from build123d import *

# Parameters (mm, degrees)
SKETCH_1_R      = 2.5
EXTRUDE_1_DEPTH = 80
SKETCH_2_R      = 2
EXTRUDE_2_DEPTH = 5
EXTRUDE_START   = 5
SKETCH_3_R      = 2
EXTRUDE_3_DEPTH = 5


with BuildPart() as part:
    # 草图1 → 凸台-拉伸1 (new body)
    with BuildSketch(Plane.XY):
        with Locations((-0.6401844, 5.281521297)):
            Circle(SKETCH_1_R)
    extrude(amount=EXTRUDE_1_DEPTH)

    # 草图2 → 凸台-拉伸2 (add)
    with BuildSketch(Plane.XY.offset(80)):
        with Locations((-0.6401844, 5.281521297)):
            Circle(SKETCH_2_R)
    extrude(amount=EXTRUDE_2_DEPTH)

    # 草图3 → 凸台-拉伸3 (add)
    with BuildSketch(Plane(origin=(0, 0, 0), x_dir=(-1, 0, 0), z_dir=(0, 0, -1)).offset(EXTRUDE_START)):
        with Locations(Location((0.6401844, 5.281521297, 0), (0, 0, 180))):
            Circle(SKETCH_3_R)
    extrude(amount=-EXTRUDE_3_DEPTH)


solid = part.part
Geometry: final body of the model. Coordinates: model frame, mm. A direction names the side the tool comes from. Give positions to 0.01 mm unless a question says otherwise; leave off trailing zeros. Write each loop counter-clockwise with the first axis right and the second up, starting at its lowest first coordinate (ties: lowest second). Pieces come first, ordered by that corner, then holes.
(1) First-contact query: P1, Ø2, axis at x = -2.5, z = 54.5, coming from the -Y side; P2, Ø1.5, axis at x = -2.5, z = 22, coming from the -Y side; P3, Ø1, axis at x = -1.5, z = 43.5, coming from the -Y side. Flat tips, straight axial feed; report the tip coordinate or a pass-through.
(2) Cut plane C-C, the plane z = 27. Return loops of the section in (x, y).
(3) Ray query, line 1 (X direction, y = 3.8, z = 61); line 2 (Z direction, x = -1.75, y = 7.05); line 3 (Y direction, x = 0.85, z = 57). Return the intervals inside material, ascending.
(4) Cut plane A-A, the plane x = -0.25. Return loops of the section in (y, z).
(5) Cut plane B-B, the plane y = 4.1. Return loops of the section in (x, z), then the cut area to 3 significant figures.
(6) Access query for faces 1 (the flat face through (-1, 5, 85)), 2 (the flat face through (-2, 7, 80)), 3 (the cylindrical face through (0.283, 7.056, -2.535)). Directions: +Z, -Z, +X, -X, +Y, -Y. A direction counts if a zero-diameter tool reaches every point of the face in a straight line with its end or side. Return the directions, or none.
Values follow:
1. P1: stops at y = 2.93
1. P2: stops at y = 3.04
1. P3: stops at y = 2.81
2. outline: circle Ø5 at (-0.64, 5.28)
3. line 1: x = -2.65 to 1.37
3. line 2: z = 0 to 80
3. line 3: y = 3.27 to 7.29
4. outline: (2.81, 0) - (3.32, 0) - (3.32, -5) - (7.24, -5) - (7.24, 0) - (7.75, 0) - (7.75, 80) - (7.24, 80) - (7.24, 85) - (3.32, 85) - (3.32, 80) - (2.81, 80) - close
5. outline: (-2.84, 0) - (-2.25, 0) - (-2.25, -5) - (0.97, -5) - (0.97, 0) - (1.56, 0) - (1.56, 80) - (0.97, 80) - (0.97, 85) - (-2.25, 85) - (-2.25, 80) - (-2.84, 80) - close
5. area: 385 mm2
6. face 1: +Z, +X, -X, +Y, -Y
6. face 2: +Z
6. face 3: -Z
